Geometry: final body of the model. Coordinates: model frame, mm. Face numbers are marked on the shaded views. Give positions to 0.01 mm unless a question says otherwise; leave off trailing zeros. Order: outer loops, then holes, each group sorted by start corner. A loop starts at its lowest first (then second) coordinate and runs counter-clockwise, first axis right, second up. Notation, with made-up numbers: M 74.25,86.5 L 116.25,86.5 A15 cw 116.25,110.5 Z; hole C 25,52 d9. An arc over 180 degrees is marked long. Write item = value, one per line. Start each with the question number.
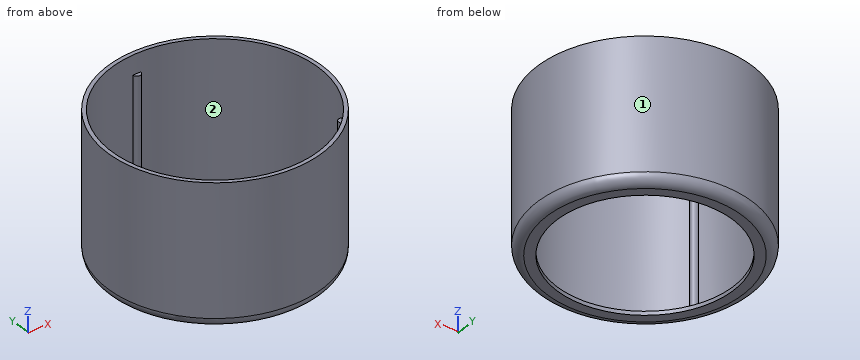
from build123d import *

# Parameters (mm, degrees)
F0_R     = 55
F0_R_2   = 45
F1_DEPTH = 2
F2_R     = 55
F2_R_2   = 53
F3_DEPTH = 70
F5_DEPTH = 60
F6_R     = 5


with BuildPart() as f1:
    # F0 (on Top) → F1 (new body)
    with BuildSketch(Plane.XY):
        Circle(F0_R)
        Circle(F0_R_2, mode=Mode.SUBTRACT)
    extrude(amount=F1_DEPTH)

    # F2 (on face) → F3 (join)
    with BuildSketch(Plane.XY.offset(2)):
        Circle(F2_R)
        Circle(F2_R_2, mode=Mode.SUBTRACT)
    extrude(amount=F3_DEPTH)

    # F4 (on face) → F5 (join, through all)
    with BuildSketch(Plane.XY.offset(2)):
        with BuildLine():
            ThreePointArc((1.9996439697, 52.9622641509), (0, 53), (-1.9996439697, 52.9622641509))
            ThreePointArc((-1.9996439697, 52.9622641509), (0, 51), (1.9996439697, 52.9622641509))
        make_face()
        with BuildLine():
            ThreePointArc((44.8668442118, -28.2128745518), (45.8993464006, -26.5), (46.8664881815, -24.7493895992))
            ThreePointArc((46.8664881815, -24.7493895992), (44.167295593, -25.5), (44.8668442118, -28.2128745518))
        make_face()
        with BuildLine():
            ThreePointArc((-44.8668442118, -28.2128745518), (-44.167295593, -25.5), (-46.8664881815, -24.7493895992))
            ThreePointArc((-46.8664881815, -24.7493895992), (-45.8993464006, -26.5), (-44.8668442118, -28.2128745518))
        make_face()
    extrude(amount=F5_DEPTH)

    # F6
    f6_edges = [f1.edges().sort_by_distance(p)[0] for p in [
        (-55, 0, 0),
    ]]
    fillet(f6_edges, radius=F6_R)


solid = f1.part
1) Cut plane B-B (y = 0). Return loops of the section in (x, z), plus the area to 3 significant figures.
2) Cut plane D-D (z = 63.5). Return loops of the section in (x, y), plus the area to 3 significant figures.
3) Ray query, L1, parallel to Y at x = -10, z = 49.5; L2, parallel to Y at x = -0.5, z = 13.5; L3, parallel to X at y = 29, z = 21. Return the intervals inside material, ascending.
4) Cut plane C-C (z = 44.5). Return loops of the section in (x, y), plus the area to 3 significant figures.
5) Cut plane A-A (x = 0). Return loops of the section in (y, z).
6) Pin query (flat end, axial travel): pin 1 Ø0.9 at (x, y) = (45, -25.5) entering from +Z; pin 2 Ø10 at (x, z) = (-27.5, 16) entering from -Y; pin 3 Ø1.5 at (x, z) = (-30, 12) entering from -Y; pin 4 Ø2.5 at (x, y) = (-45.5, -26) entering from +Z. Return the tip coordinate at first contact, or that it passes through.
7) Draft query along X for the marked faces 1 and 2. Return one class per face: pulls with the +X half, pulls with the -X half, needs draft (parallel to the pull), parting line crosses it, or undercut.
Reply:
q1.outline = M -55,5 A5 ccw -50,0 L -45,0 L -45,2 L -53,2 L -53,72 L -55,72 Z; M 45,0 L 50,0 A5 ccw 55,5 L 55,72 L 53,72 L 53,2 L 45,2 Z
q1.area = 309 mm²
q2.outline = C 0,0 d110; hole C 0,0 d106
q2.area = 679 mm²
q3.L1 = -54.08 to -52.05, 52.05 to 54.08
q3.L2 = -55 to -53, 51.06 to 55
q3.L3 = -46.73 to -44.36, 44.36 to 46.73
q4.outline = C 0,0 d110; hole M -46.87,-24.75 A2 cw -44.87,-28.21 A53 ccw 44.87,-28.21 A2 cw 46.87,-24.75 A53 ccw 2,52.96 A2 cw -2,52.96 A53 ccw Z
q4.area = 697 mm²
q5.outline = M -55,5 A5 ccw -50,0 L -45,0 L -45,2 L -53,2 L -53,72 L -55,72 Z; M 45,0 L 50,0 A5 ccw 55,5 L 55,72 L 53,72 L 53,62 L 51,62 L 51,2 L 45,2 Z
q6.pin_1 = 62
q6.pin_2 = -50.19
q6.pin_3 = -46.58
q6.pin_4 = 72
q7.face_1 = parting line crosses it
q7.face_2 = undercut
